Verification items for the finished model (mm, model axes). A direction names the side the tool comes from. Give positions to 0.01 mm unless a question says otherwise; leave off trailing zeros. Write each loop counter-clockwise with the first axis right and the second up, starting at its lowest first coordinate (ties: lowest second). Pieces come first, ordered by that corner, then holes. Notation, with made-up numbers: (-18.75, 4) - (13.25, 4) arc R32 ccw to (13.25, 41) - close; hole circle Ø1 at (-29.5, 44). An arc over 180 degrees is marked (long way). Put each result on its own line as item: value.
from build123d import *

# Parameters (mm, degrees)
SKETCH1_W           = 20
SKETCH1_H           = 4.8
BOSS_EXTRUDE1_DEPTH = 5
FILLET1_R           = 10
SKETCH2_R           = 2.1
CUT_EXTRUDE1_DEPTH  = 5


with BuildPart() as part:
    # Sketch1 → Boss-Extrude1 (new body)
    with BuildSketch(Plane.XY):
        Polygon((125.000000001, -10), (-124.999999999, -10), (-124.999999999, 20), (-129.999999999, 20), (-129.999999999, 40), (-124.999999999, 40), (-124.999999999, 130), (-129.999999999, 130), (-129.999999999, 150), (-124.999999999, 150), (-124.999999999, 180), (-74.999999999, 180), (-50, 60), (50, 60), (75.000000001, 180), (125.000000001, 180), (125.000000001, 150), (130.000000001, 150), (130.000000001, 130), (125.000000001, 130), (125.000000001, 40), (130.000000001, 40), (130.000000001, 20), (125.000000001, 20), align=None)
        with Locations((85.000000001, -2.5)):
            Rectangle(SKETCH1_W, SKETCH1_H, mode=Mode.SUBTRACT)
        with Locations((-84.999999999, -2.5)):
            Rectangle(SKETCH1_W, SKETCH1_H, mode=Mode.SUBTRACT)
    extrude(amount=BOSS_EXTRUDE1_DEPTH)

    # Fillet1
    fillet1_edges = [part.edges().sort_by_distance(p)[0] for p in [
        (-50, 60, 2.5),
        (50, 60, 2.5),
    ]]
    fillet(fillet1_edges, radius=FILLET1_R)

    # Sketch2 → Cut-Extrude1 (cut)
    with BuildSketch(Plane.XY.offset(5)):
        with Locations((-109.999999999, 15)):
            Circle(SKETCH2_R)
        with Locations((110.000000001, 15)):
            Circle(SKETCH2_R)
        with Locations((110.000000001, 165)):
            Circle(SKETCH2_R)
        with Locations((-109.999999999, 165)):
            Circle(SKETCH2_R)
    extrude(amount=-CUT_EXTRUDE1_DEPTH, mode=Mode.SUBTRACT)


solid = part.part
Q1. Set-up check for faces 1 (the face through (-63.5, 124.8, 2.5)), 2 (the face through (128, 20, 2)), 3 (the face through (127, 40, 2)): record each of +Z, -Z, +X, -X, +Y, -Y from which the full face is reachable in a straight line by a thin tool's end or side.
Answers follow:
face 1: +Z, -Z, +Y
face 2: +Z, -Z, +X, -Y
face 3: +Z, -Z, +X
Q2. Go/stop test with flat-tipped pins: pin 1 Ø1.5 at (y, z) = (11.5, 1.5) entering from -X; pin 2 Ø1.5 at (y, z) = (9.5, 1.5) entering from +X; pin 3 Ø3.5 at (x, y) = (-110, 165) entering from +Z; pin 4 Ø2.5 at (x, z) = (-127.5, 3.5) entering from -Y. Record where each tip stops, or that it passes through.
Answers follow:
pin 1: stops at x = -125
pin 2: stops at x = 125
pin 3: passes through
pin 4: stops at y = 20
Q3. Section check D-D, the plane x = 27.5. Record the cut outline in (y, z).
Answers follow:
outline: (-10, 0) - (60, 0) - (60, 5) - (-10, 5) - close
Q4. Section check B-B, the plane y = 82.5. Record the cut outline in (x, z), plus the area to 3 significant figures.
Answers follow:
outline: (-125, 0) - (-54.69, 0) - (-54.69, 5) - (-125, 5) - close; (54.69, 0) - (125, 0) - (125, 5) - (54.69, 5) - close
area: 703 mm2
Q5. Section check A-A, the plane x = 84. Record the cut outline in (y, z).
Answers follow:
outline: (-10, 0) - (-4.9, 0) - (-4.9, 5) - (-10, 5) - close; (-0.1, 0) - (180, 0) - (180, 5) - (-0.1, 5) - close
Q6. Section check C-C, the plane z = 1.15. Give the number of separate pieces and of enclosed holes in the cut face, plus the area to 3 significant figures.
Answers follow:
separate pieces: 1
enclosed holes: 6
area: 32,700 mm2
Q7. Release check for a two-part mould opening along X. For faces 4 (the face through (85, -0.1, 2)), 5 (the face through (125, 165, 2)), 6 (the face through (-1, 60, 2)), 7 (the face through (-130, 30, 2)) record: released by +X, released by -X, zero draft, split by the parting line, or undercut.
Answers follow:
face 4: undercut
face 5: released by +X
face 6: undercut
face 7: released by -X
Q8. Scan lines: line 1 along Y through (x, z) = (110, 2.15); line 2 along X through (y, z) = (16.5, 2.7); line 3 along X through (y, z) = (165, 1.7) (3 decimals). Record each from-to range of solid material in increasing order.
Answers follow:
line 1: y = -10 to 12.9, 17.1 to 162.9, 167.1 to 180
line 2: x = -125 to -111.47, -108.53 to 108.53, 111.47 to 125
line 3: x = -125 to -112.1, -107.9 to -71.875, 71.875 to 107.9, 112.1 to 125
